Autodesk Inventor part; units mm, degrees
ref_plane "YZ Plane" through (0, 0, 0) normal (1, 0, 0) x (0, 1, 0)
ref_plane "XZ Plane" through (0, 0, 0) normal (0, 1, 0) x (-1, 0, 0)
ref_plane "XY Plane" through (0, 0, 0) normal (0, 0, 1) x (1, 0, 0)
sketch "Sketch1" plane through (0, 0, 0) normal (0, 0, 1) x (1, 0, 0)
  circle A0 centre (0, 0) radius 4
  line L0 (4, 0) -> (2, -3.4641)
  line L1 (2, -3.4641) -> (-2, -3.4641)
  line L2 (-2, -3.4641) -> (-4, 0)
  line L3 (-4, 0) -> (-2, 3.4641)
  line L4 (-2, 3.4641) -> (2, 3.4641)
  line L5 (2, 3.4641) -> (4, 0)
  dimension "d0" = 8
extrude "Extrusion1" add sketch "Sketch1" against normal blind 5
sketch "Sketch2" plane through (0, 0, -5) normal (0, 0, -1) x (-1, 0, 0)
  circle A0 centre (0, 0) radius 4
  line L0 (-4, 4) -> (4, 4)
  line L1 (4, 4) -> (4, -4)
  line L2 (4, -4) -> (-4, -4)
  line L3 (-4, -4) -> (-4, 4)
  point P0 (-4, 0)
extrude "Extrusion2" add sketch "Sketch2" along normal blind 8
sketch "Sketch3" plane through (0, 0, 0) normal (0, 0, 1) x (1, 0, 0)
  line L0 (4, -2.3094) -> (0, -4.6188)
  line L1 (-2.75, -2.75) -> (-2.75, 2.75)
  line L2 (-2.75, 2.75) -> (2.75, 2.75)
  line L3 (2.75, 2.75) -> (2.75, -2.75)
  line L4 (2.75, -2.75) -> (-2.75, -2.75)
  point P0 (0, 0)
  point P1 (0, -2.75)
  dimension "d7" = 5.5
  dimension "d8" = 5.5
extrude "Extrusion3" add sketch "Sketch3" along normal blind 9
mirror "Mirror1" about plane through (0, 0, -13) normal (0, 0, -1) of "Extrusion1", "Extrusion2", "Extrusion3"
scale "Scale1" factors (0.5, 0.5, 0.5) then translate (0, 2, -6.5) bodies 1
properties part number "GearAxis"
Design review of the part built by this model. Coordinates are the model's own, in mm. A direction names the side the tool comes from. Give positions to 0.01 mm unless a question says otherwise; leave off trailing zeros. Write each loop counter-clockwise with the first axis right and the second up, starting at its lowest first coordinate (ties: lowest second). Pieces come first, ordered by that corner, then holes. Notation, with made-up numbers: M 9.5,-18 L 13.5,-18 A20 ccw 13.5,17 Z; hole C 18.25,35.5 d4. An arc over 180 degrees is marked long. Return JSON: item names as keys, results as strings. Group by question number.
Item 1: Clearance check with flat-ended pins moving along their axes: pin 1 Ø1.4 at (x, z) = (0.5, -22.5) entering from +Y (3 decimals); pin 2 Ø2 at (x, y) = (-1.5, 1.5) entering from -Z; pin 3 Ø2 at (y, z) = (2, -4.5) entering from -X (3 decimals); pin 4 Ø0.8 at (y, z) = (2, -22.5) entering from +X (3 decimals). State where each tip first meets the part, or that it passes through.
Item 2: Take a section at A-A (y = 3.7). Give the boundary of the cut face in (x, z).
Item 3: Tool access review of faces 1 (the flat face through (1.6, 0.4, -17)), 2 (the flat face through (0, 0.625, -22)), 3 (the flat face through (1.6, 3.5, -9)), 4 (the flat face through (0, 3.375, -4)), 5 (the flat face through (-1.6, 0.5, -17)): name each direction out of +Z, -Z, +X, -X, +Y, -Y from which nothing blocks a thin tool from reaching the whole face with its end or side.
Item 4: Take a section at B-B (x = 1.65). Give the boundary of the cut face in (y, z), plus the area to 3 significant figures.
Item 5: Take a section at C-C (z = -21). Give the boundary of the cut face in (x, y) (3 decimals), plus the area to 3 significant figures.
Item 6: Take a section at D-D (x = -0.35). Give the boundary of the cut face in (y, z) (3 decimals).
Item 7: Wall thickness on line 1 along Y through (x, z) = (-0.5, -21.5) (3 decimals); line 2 along Z through (x, y) = (-0.55, 3.75); line 3 along Z through (x, y) = (-1.25, 0.35): over which ranges is each line inside the solid? List them lowest first.
Return value:
{
 "1": {"pin 1": "stops at y = 3.375", "pin 2": "stops at z = -24", "pin 3": "stops at x = -1.375", "pin 4": "stops at x = 1.375"},
 "2": {"outline": "M -2,-17 L -1.05,-17 L -1.05,-19.5 L 1.05,-19.5 L 1.05,-17 L 2,-17 L 2,-9 L 1.05,-9 L 1.05,-6.5 L -1.05,-6.5 L -1.05,-9 L -2,-9 Z"},
 "3": {"face 1": "-Z, +X, -Y", "face 2": "-Z, +X, -X, -Y", "face 3": "+Z, +X, +Y", "face 4": "+Z, +X, -X, +Y", "face 5": "-Z, -X, -Y"},
 "4": {"outline": "M 0,-17 L 0.87,-17 L 0.87,-19.5 L 3.13,-19.5 L 3.13,-17 L 4,-17 L 4,-9 L 3.13,-9 L 3.13,-6.5 L 0.87,-6.5 L 0.87,-9 L 0,-9 Z", "area": "43.3 mm2"},
 "5": {"outline": "M -1.375,0.625 L 1.375,0.625 L 1.375,3.375 L -1.375,3.375 Z", "area": "7.56 mm2"},
 "6": {"outline": "M 0,-17 L 0.031,-17 L 0.031,-19.5 L 0.625,-19.5 L 0.625,-24 L 3.375,-24 L 3.375,-19.5 L 3.969,-19.5 L 3.969,-17 L 4,-17 L 4,-9 L 3.969,-9 L 3.969,-6.5 L 3.375,-6.5 L 3.375,-2 L 0.625,-2 L 0.625,-6.5 L 0.031,-6.5 L 0.031,-9 L 0,-9 Z"},
 "7": {"line 1": "y = 0.625 to 3.375", "line 2": "z = -19.5 to -6.5", "line 3": "z = -17 to -9"}
}
